```python
from build123d import *

# Parameters (mm, degrees)
BOSS_EXTRUDE1_DEPTH = 20
SKETCH3_R           = 2.65
CUT_EXTRUDE1_DEPTH  = 182.148333213
SKETCH4_R           = 2.65
CUT_EXTRUDE2_DEPTH  = 201.997512422
SKETCH5_R           = 5.5
CUT_EXTRUDE3_DEPTH  = 198.511484318
SKETCH6_R           = 5.5
CUT_EXTRUDE4_DEPTH  = 178.272403558


with BuildPart() as part:
    # Sketch2 → Boss-Extrude1 (new body)
    with BuildSketch(Plane(origin=(0, 0, 0), x_dir=(0, 0, -1), z_dir=(1, 0, 0))):
        Polygon((0, 0), (-111.421356237, 111.421356237), (-111.421356237, 141.421356237), (30, 0), align=None)
    extrude(amount=BOSS_EXTRUDE1_DEPTH)

    # Sketch3 → Cut-Extrude1 (cut, through all)
    with BuildSketch(Plane.XZ):
        with Locations(Location((10, -15, 0), (0, 0, 270))):
            Circle(SKETCH3_R)
    extrude(amount=-CUT_EXTRUDE1_DEPTH, mode=Mode.SUBTRACT)

    # Sketch4 → Cut-Extrude2 (cut, through all)
    with BuildSketch(Plane.XY.offset(111.421356237)):
        with Locations((10, 126.421356237)):
            Circle(SKETCH4_R)
    extrude(amount=-CUT_EXTRUDE2_DEPTH, mode=Mode.SUBTRACT)

    # Sketch5 → Cut-Extrude3 (cut, through all)
    with BuildSketch(Plane.XY.offset(106.421356237)):
        with Locations((10, 126.421356237)):
            Circle(SKETCH5_R)
    extrude(amount=-CUT_EXTRUDE3_DEPTH, mode=Mode.SUBTRACT)

    # Sketch6 → Cut-Extrude4 (cut, through all)
    with BuildSketch(Plane(origin=(0, 5, 0), x_dir=(-1, 0, 0), z_dir=(0, -1, 0))):
        with Locations(Location((-10, 15, 0), (0, 0, 90))):
            Circle(SKETCH6_R)
    extrude(amount=-CUT_EXTRUDE4_DEPTH, mode=Mode.SUBTRACT)


solid = part.part
```
Geometry: final body of the model. Coordinates: model frame, mm. A direction names the side the tool comes from. Round coordinates to 2 decimals unless told otherwise and drop trailing zeros. Loops run counter-clockwise (first coordinate to the right, second up) from the corner with the lowest first, then second, coordinate; pieces in that order, holes last. Notation, with made-up numbers: (11.25, -28.5) -> (16.25, -28.5) arc R31 ccw to (16.25, 9.5) -> close; hole circle Ø9 at (57, 56.25). An arc over 180 degrees is marked (long way). Use one line per item in the form item = value.
Item 1: Access query for faces 4 (the flat face through (9, 5, -12)), 5 (the flat face through (7, 125, 106.421)), 6 (the cylindrical face through (8.99, 2.46, -17.45)). Directions: +Z, -Z, +X, -X, +Y, -Y. A direction counts if a zero-diameter tool reaches every point of the face in a straight line with its end or side. Return the directions, or none.
Evaluation:
face_4 = +Y
face_5 = -Z
face_6 = +Y, -Y
Item 2: Cut plane A-A on z = -15. Output: boundary loops of the cut face in (x, y), then the cut area to 4 significant figures.
Evaluation:
outline = (0, 0) -> (7.35, 0) -> (7.35, 5) -> (4.5, 5) -> (4.5, 15) -> (0, 15) -> close; (12.65, 0) -> (20, 0) -> (20, 15) -> (15.5, 15) -> (15.5, 5) -> (12.65, 5) -> close
area = 163.5 mm2
Item 3: Cut plane C-C on z = 38. Output: boundary loops of the cut face in (x, y).
Evaluation:
outline = (0, 38) -> (20, 38) -> (20, 68) -> (0, 68) -> close
Item 4: Draft query along X for faces 1 (the flat face through (10, 72, 42)), 2 (the flat face through (0, 61, 46)), 3 (the cylindrical face through (10.242, 11.006, -9.505)). Return one class per face: released by +X, released by -X, zero draft, split by the parting line, or undercut.
Evaluation:
face_1 = zero draft
face_2 = released by -X
face_3 = undercut
Item 5: Cut plane D-D on y = 71.5. Output: boundary loops of the cut face in (x, z), then the cut area to 3 significant figures.
Evaluation:
outline = (0, 41.5) -> (20, 41.5) -> (20, 71.5) -> (0, 71.5) -> close
area = 600 mm2
Item 6: Material intervals for probe 1 along X at (y, z) = (11, -15); probe 2 along X at (y, z) = (1.85, -15); probe 3 along Z at (x, y) = (17.5, 116.5), sorted ascending.
Evaluation:
probe_1 = 0 to 4.5, 15.5 to 20
probe_2 = 0 to 7.35, 12.65 to 20
probe_3 = 86.5 to 111.42
Item 7: Cut plane B-B on x = 10. Output: boundary loops of the cut face in (y, z).
Evaluation:
outline = (0, -30) -> (9.5, -20.5) -> (5, -20.5) -> (5, -17.65) -> (0, -17.65) -> close; (0, -12.35) -> (5, -12.35) -> (5, -9.5) -> (20.5, -9.5) -> (120.92, 90.92) -> (120.92, 106.42) -> (123.77, 106.42) -> (123.77, 111.42) -> (111.42, 111.42) -> (0, 0) -> close; (129.07, 106.42) -> (131.92, 106.42) -> (131.92, 101.92) -> (141.42, 111.42) -> (129.07, 111.42) -> close
Item 8: Contact query for flat-ended pins moving along their axis: pin 1 Ø5.5 at (x, y) = (9.5, 127) entering from -Z; pin 2 Ø4 at (x, y) = (7, 120) entering from -Z; pin 3 Ø5 at (x, z) = (12, 28.5) entering from +Y. Output: stop coordinate, or through.
Evaluation:
pin_1 = 106.42
pin_2 = 88
pin_3 = 61
